Verification items for the finished model (mm, model axes). A direction names the side the tool comes from. Round coordinates to 2 decimals unless told otherwise and drop trailing zeros. Write each loop counter-clockwise with the first axis right and the second up, starting at its lowest first coordinate (ties: lowest second). Pieces come first, ordered by that corner, then holes.
Autodesk Inventor part; units mm, degrees
ref_plane "Work Plane1" through (0, 0, 45) normal (0, 0, -1) x (-1, 0, 0)
ref_plane "YZ Plane" through (0, 0, 0) normal (1, 0, 0) x (0, 1, 0)
ref_plane "XZ Plane" through (0, 0, 0) normal (0, 1, 0) x (-1, 0, 0)
sketch "Sketch1" plane through (0, 0, 0) normal (0, 0, 1) x (1, 0, 0)
  line L0 (0, 0) -> (-45, 0)
  line L1 (-45, 0) -> (-45, 45)
  line L2 (-45, 45) -> (0, 45)
  line L3 (0, 45) -> (0, 0)
  line L4 (-2, 45) -> (-2, 0)
  line L5 (-45, 2) -> (-2, 2)
  line L6 (-2, 45) -> (-45, 45)
  line L7 (-45, 45) -> (-45, 43)
  line L8 (-45, 43) -> (-2, 43)
  line L9 (-2, 43) -> (-2, 45)
  line L10 (-45, 43) -> (-43, 43)
  line L11 (-43, 43) -> (-43, 28)
  line L12 (-43, 28) -> (-45, 28)
  line L13 (-45, 28) -> (-45, 43)
  dimension "d0" = 45
  dimension "d1" = 45
  dimension "d2" = 2
  dimension "d3" = 2
  dimension "d17" = 2
  dimension "d18" = 2
  dimension "d19" = 15
extrude "Extrusion1" add sketch "Sketch1" along normal blind 90 contours L0 L4 L2 L3 | L0 L1 L5 L4
sketch "Sketch2" plane through (0, 0, 90) normal (0, 0, 1) x (1, 0, 0)
  line L0 (-45, 0) -> (0, 0)
  line L1 (0, 0) -> (-30, 0)
  line L2 (-30, 0) -> (-30, 30)
  line L3 (-30, 30) -> (0, 30)
  line L4 (0, 30) -> (0, 0)
  line L5 (0, 0) -> (-21.8882, 0)
  line L6 (-21.8882, 0) -> (0, 30)
  dimension "d6" = 30
  dimension "d7" = 30
  dimension "d8" = 30
extrude "Extrusion2" add sketch "Sketch2" against normal blind 2 contours L6 L4 L0
ref_plane "Work Plane1" through (0, 0, 45) normal (0, 0, -1) x (-1, 0, 0)
sketch "Sketch3" plane through (0, 0, 0) normal (1, 0, 0) x (0, 0, -1)
  line L0 (-80, 30) -> (-10, 30)
  line L1 (-10, 30) -> (-10, -10)
  line L2 (-10, -10) -> (-80, -10)
  line L3 (-80, -10) -> (-80, 30)
  line L4 (0, 45) -> (-90, 45)
  line L5 (0, 0) -> (0, 45)
  dimension "d11" = 70
  dimension "d12" = 40
  dimension "d13" = 15
  dimension "d14" = 10
extrude "Extrusion3" cut sketch "Sketch3" against normal blind 20
extrude "Extrusion4" add sketch "Sketch1" along normal blind 90 contours L4 L8 L1 L2 | L1 L8 L11 L12
properties part number "belt_holder"
Q1. Tool access check on faces 4 (the flat face through (-1, 30, 45)), 5 (the flat face through (-11.343, 14.453, 89.014)), 6 (the flat face through (-23, 43, 44)). Record the directions out of +Z, -Z, +X, -X, +Y, -Y that give a thin tool (end or side, any length) a straight path to the whole face; none if there is none.
Recorded:
face 4: +X, -Y
face 5: +Z, -Z, -X
face 6: +Z, -Z
Q2. Sectioned sample at D-D (x = -14.5). Enter the section's corners in (y, z).
Recorded:
outline: (0, 0) - (2, 0) - (2, 10) - (0, 10) - close; (0, 80) - (2, 80) - (2, 88) - (10.13, 88) - (10.13, 90) - (0, 90) - close; (43, 0) - (45, 0) - (45, 90) - (43, 90) - close
Q3. Release check for a two-part mould opening along Y. For faces 1 (the flat face through (-1.8, 9.5, 10)), 2 (the flat face through (-27, 0, 44)), 3 (the flat face through (-44, 28, 44)) record: released by +Y, released by -Y, zero draft, split by the parting line, or undercut.
Recorded:
face 1: zero draft
face 2: released by -Y
face 3: undercut
Q4. Sectioned sample at C-C (x = -34.5). Enter the section's corners in (y, z), plus the area to 3 significant figures.
Recorded:
outline: (0, 0) - (2, 0) - (2, 90) - (0, 90) - close; (43, 0) - (45, 0) - (45, 90) - (43, 90) - close
area: 360 mm2
Q5. Material ranges on line 1 along Y through (x, z) = (-22.5, 32); line 2 along X through (y, z) = (29, 67); line 3 along Y through (x, z) = (-16, 20), recorded low to high.
Recorded:
line 1: y = 0 to 2, 43 to 45
line 2: x = -45 to -43
line 3: y = 43 to 45
Q6. Depth check by flat-ended pin: P1, Ø1, axis at x = -1, z = 56, coming from the -Y side; P2, Ø9, axis at x = -10.5, y = 19.5, coming from the -Z side; P3, Ø0.6, axis at y = 1, z = 46.5, coming from the +X side. Enter the tip coordinate at first touch or a pass-through.
Recorded:
P1: stops at y = 30
P2: stops at z = 88
P3: stops at x = -20
Q7. Sectioned sample at A-A (y = 34.5). Enter the section's corners in (x, z), plus the area to 3 significant figures.
Recorded:
outline: (-45, 0) - (-43, 0) - (-43, 90) - (-45, 90) - close; (-2, 0) - (0, 0) - (0, 90) - (-2, 90) - close
area: 360 mm2
Q8. Sectioned sample at B-B (z = 29). Enter the section's corners in (x, y), plus the area to 3 significant figures.
Recorded:
outline: (-45, 0) - (-20, 0) - (-20, 2) - (-45, 2) - close; (-45, 28) - (-43, 28) - (-43, 43) - (-2, 43) - (-2, 30) - (0, 30) - (0, 45) - (-45, 45) - close
area: 196 mm2
